```python
from build123d import *

# Parameters (mm, degrees)
EXTRUDE_1_DEPTH     = 2
SKETCH_3_W          = 9.5
SKETCH_3_H          = 8
CUT_EXTRUDE_1_DEPTH = 1.2
SKETCH_4_W          = 5
SKETCH_4_H          = 5
CUT_EXTRUDE_2_DEPTH = 1
EXTRUDE_2_DEPTH     = 1
FILLET_1_R          = 1.6
SKETCH_6_W          = 9.5
SKETCH_6_H          = 6
SKETCH_6_W_2        = 9
SKETCH_6_W_3        = 4.6
SKETCH_6_H_2        = 8
EXTRUDE_3_DEPTH     = 2
CHAMFER_1_SIZE      = 2.5
CHAMFER_2_SIZE      = 2
FILLET_2_R          = 3
SKETCH_7_R          = 0.85
CUT_EXTRUDE_3_DEPTH = 74.33655296
SKETCH_8_R          = 1.25
CUT_EXTRUDE_4_DEPTH = 74.33655296
SKETCH_9_R          = 2.5
CUT_EXTRUDE_5_DEPTH = 0.6
FILLET_3_R          = 0.4
SKETCH_10_W         = 12.125863774
SKETCH_10_H         = 8.335254798
CUT_EXTRUDE_6_DEPTH = 0.2
EXTRUDE_4_DEPTH     = 1


with BuildPart() as part:
    # 草图2 → 凸台-拉伸1 (new body)
    with BuildSketch(Plane(origin=(0, 0, 0), x_dir=(1, 0, 0), z_dir=(0, 1, 0))):
        Polygon((40, 41), (44.5, 41), (44.5, 50), (53.5, 50), (53.5, 0), (0, 0), (0, 8), (40, 8), align=None)
    extrude(amount=EXTRUDE_1_DEPTH)

    # 草图3 → 切除-拉伸1 (cut)
    with BuildSketch(Plane.XZ):
        with Locations((11, -4)):
            Rectangle(SKETCH_3_W, SKETCH_3_H)
    extrude(amount=-CUT_EXTRUDE_1_DEPTH, mode=Mode.SUBTRACT)

    # 草图4 → 切除-拉伸2 (cut)
    with BuildSketch(Plane.XZ):
        with Locations((20.9, -2.5)):
            Rectangle(SKETCH_4_W, SKETCH_4_H)
    extrude(amount=-CUT_EXTRUDE_2_DEPTH, mode=Mode.SUBTRACT)

    # 草图5 → 凸台-拉伸2 (add)
    with BuildSketch(Plane.XY):
        Polygon((0, 0), (0, -2), (6.25, -2), (6.25, 0), (6.25, 1.2), (15.75, 1.2), (15.75, -2), (18.4, -2), (18.4, 1), (23.4, 1), (23.4, 0), (23.4, -2), (27.9, -2), (27.9, 0), (42.9, 0), (42.9, -2), (53.5, -2), (53.5, 0), (53.5, 2), (0, 2), align=None)
    extrude(amount=EXTRUDE_2_DEPTH)

    # 圆角1
    fillet_1_edges = [part.edges().sort_by_distance(p)[0] for p in [
        (15.75, 1.2, -3.5),
        (6.25, 1.2, -3.5),
    ]]
    fillet(fillet_1_edges, radius=FILLET_1_R)

    # 草图6 → 凸台-拉伸3 (add)
    with BuildSketch(Plane.XZ):
        with Locations((48.75, -3)):
            Rectangle(SKETCH_6_W, SKETCH_6_H)
        with Locations((49, -47)):
            Rectangle(SKETCH_6_W_2, SKETCH_6_H)
        with Locations((2.3, -4)):
            Rectangle(SKETCH_6_W_3, SKETCH_6_H_2)
    extrude(amount=EXTRUDE_3_DEPTH)

    # 倒角1
    chamfer_1_edges = [part.edges().sort_by_distance(p)[0] for p in [
        (53.5, 0, 1),
    ]]
    chamfer(chamfer_1_edges, length=CHAMFER_1_SIZE)

    # 倒角2
    chamfer_2_edges = [part.edges().sort_by_distance(p)[0] for p in [
        (48.75, 0, -6),
        (49, 0, -44),
    ]]
    chamfer(chamfer_2_edges, length=CHAMFER_2_SIZE - 0.0001)  # a hair under: the kernel refuses the full size

    # 圆角2
    fillet_2_edges = [part.edges().sort_by_distance(p)[0] for p in [
        (0, 0, -8),
        (40, 1, -8),
        (40, 1, -41),
        (44.5, 0, -50),
    ]]
    fillet(fillet_2_edges, radius=FILLET_2_R)

    # 草图7 → 切除-拉伸3 (cut, through all)
    with BuildSketch(Plane.XZ.offset(2)):
        with Locations(Location((47, -3, 0), (0, 0, 270))):
            Circle(SKETCH_7_R)
        with Locations(Location((47, -47, 0), (0, 0, 270))):
            Circle(SKETCH_7_R)
        with Locations(Location((3, -3, 0), (0, 0, 270))):
            Circle(SKETCH_7_R)
    extrude(amount=-CUT_EXTRUDE_3_DEPTH, mode=Mode.SUBTRACT)

    # 草图8 → 切除-拉伸4 (cut, through all)
    with BuildSketch(Plane(origin=(0, 2, 0), x_dir=(1, 0, 0), z_dir=(0, 1, 0))):
        with Locations(Location((44, 37.5, 0), (0, 0, 270))):
            Circle(SKETCH_8_R)
    extrude(amount=-CUT_EXTRUDE_4_DEPTH, mode=Mode.SUBTRACT)

    # 草图9 → 切除-拉伸5 (cut)
    with BuildSketch(Plane.XZ):
        with Locations(Location((44, -37.5, 0), (0, 0, 270))):
            Circle(SKETCH_9_R)
    extrude(amount=-CUT_EXTRUDE_5_DEPTH, mode=Mode.SUBTRACT)

    # 圆角3
    fillet_3_edges = [part.edges().sort_by_distance(p)[0] for p in [
        (51, 0, 1),
    ]]
    fillet(fillet_3_edges, radius=FILLET_3_R)

    # 草图10 → 切除-拉伸6 (cut)
    with BuildSketch(Plane.XZ.offset(2)):
        with Locations((49.021088356, -47.204499244)):
            Rectangle(SKETCH_10_W, SKETCH_10_H)
    extrude(amount=-CUT_EXTRUDE_6_DEPTH, mode=Mode.SUBTRACT)

    # 草图11 → 凸台-拉伸4 (add)
    with BuildSketch(Plane.XY.offset(1)):
        Polygon((23.4, 1), (23.4, -2), (22.8, -2), (22.8, 0), (19.3, 0), (19.3, -2), (18.4, -2), (18.4, 1), align=None)
    extrude(amount=-EXTRUDE_4_DEPTH)


solid = part.part
```
Could you check a few things on this model? Use its own coordinates, in mm. A direction names the side the tool comes from. Round coordinates to 2 decimals unless told otherwise and drop trailing zeros. Write each loop counter-clockwise with the first axis right and the second up, starting at its lowest first coordinate (ties: lowest second). Pieces come first, ordered by that corner, then holes.
(1) Suppose I cut it at A-A on z = -3. Write out the boundary of the cut face in (x, y), and give its area (3 significant figures).
Findings below:
outline: (0, -2) - (2.15, -2) - (2.15, 2) - (0, 2) - close; (3.85, -2) - (4.6, -2) - (4.6, 0) - (6.3, 0) arc R1.6 cw to (7.85, 1.2) - (14.15, 1.2) arc R1.6 cw to (15.7, 0) - (18.4, 0) - (18.4, 1) - (23.4, 1) - (23.4, 0) - (44, 0) - (44, -2) - (46.15, -2) - (46.15, 2) - (3.85, 2) - close; (47.85, -2) - (53.5, -2) - (53.5, 2) - (47.85, 2) - close
area: 106 mm2
(2) If I drill on probe 1 along X at (y, z) = (-0.15, -3); probe 2 along X at (y, z) = (-1.45, -2); probe 3 along Z at (x, y) = (47, -0.5), over which ranges is the centre line in solid material (lowest first)?
Findings below:
probe 1: x = 0 to 2.15, 3.85 to 4.6, 44 to 46.15, 47.85 to 53.5
probe 2: x = 0 to 4.6, 44 to 53.5
probe 3: z = -49.96 to -47.85, -46.15 to -42.5, -7.5 to -3.85, -2.15 to 1
(3) Suppose I cut it at B-B on x = 22. Write out the boundary of the cut face in (y, z), and give its area (3 significant figures).
Findings below:
outline: (0, -8) - (2, -8) - (2, 1) - (0, 1) - (0, 0) - (1, 0) - (1, -5) - (0, -5) - close
area: 13.0 mm2
(4) Suppose I cut it at C-C on z = -17.5. Write out the boundary of the cut face in (x, y), and give its area (3 significant figures).
Findings below:
outline: (40, 0) - (53.5, 0) - (53.5, 2) - (40, 2) - close
area: 27.0 mm2
(5) Thinking about a two-plate mould opening in X: for faces 1 (the face through (20, 1, -8)), 2 (the face through (40, 1, -24)), 3 (the face through (46.48, 0.07, -46.33)), which applies, +X half, -X half, draft (parallel to the pull), parting line (faces both ways), or undercut?
Findings below:
face 1: draft
face 2: -X half
face 3: undercut
(6) Suppose I cut it at D-D on x = 33. Write out the boundary of the cut face in (y, z), and give its area (3 significant figures).
Findings below:
outline: (0, -8) - (2, -8) - (2, 1) - (0, 1) - close
area: 18.0 mm2
(7) For pin 1 (0.8 mm diameter, centred on y = -1.5, z = 0.5, fed in from +X); pin 2 (2 mm diameter, centred on x = 47, z = -47, fed in from -Y); pin 3 (12 mm diameter, centred on x = 48, z = -20, fed in from -Y), each with a flat end and sliding along its axis, tell me the tip position at first contact or that it passes through.
Findings below:
pin 1: stops at x = 51.9
pin 2: stops at y = -1.8
pin 3: stops at y = 0
(8) Which directions (+Z, -Z, +X, -X, +Y, -Y) give clear straight access to the entire face, cutting with the end or side of a thin tool? Please do faces 4 (the face through (49, -1.8, -47)), 5 (the face through (44, -1, -3)), 6 (the face through (21.9, 0.2, 0)), 7 (the face through (6.73, 0.74, -3.44)).
Findings below:
face 4: -Z, +X, -X, -Y
face 5: -Z, -Y
face 6: -Y
face 7: +Z, -Z, -Y
